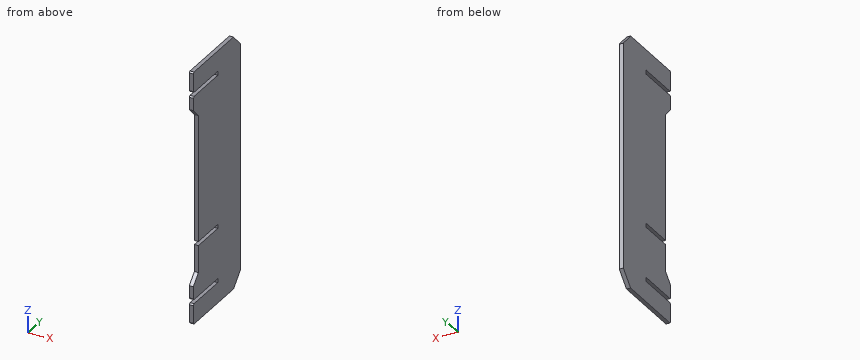
from build123d import *

# Parameters (mm, degrees)
SKETCH1_W                = 3
SKETCH1_H                = 7.073755714
SKETCH1_H_2              = 58.176244286
BOSS_EXTRUDE1_DEPTH      = 15
BOSS_EXTRUDE1_DEPTH_BACK = 171
CUT_EXTRUDE1_REACH       = 5
SKETCH2_W                = 3
SKETCH2_H                = 7.071067812
SKETCH2_H_2              = 26.692349798
CHAMFER1_SIZE            = 10
SKETCH5_W                = 3
SKETCH5_H                = 3
CUT_EXTRUDE2_DEPTH       = 1.002687902
CUT_EXTRUDE3_REACH       = 2.003
SKETCH6_W                = 3
SKETCH6_H                = 3
CHAMFER2_SIZE            = 1


with BuildPart() as part:
    # Sketch1 → Boss-Extrude1 (new body, two sides)
    with BuildSketch(Plane.XY) as boss_extrude1_sk:
        with Locations((-220.627859803, -123.051259948)):
            Rectangle(SKETCH1_W, SKETCH1_H)
        with Locations((-220.627859803, -90.426259948)):
            Rectangle(SKETCH1_W, SKETCH1_H_2)
    extrude(amount=BOSS_EXTRUDE1_DEPTH)
    extrude(boss_extrude1_sk.sketch, amount=-BOSS_EXTRUDE1_DEPTH_BACK)

    # Sketch2 → Cut-Extrude1 (cut, up to next)
    with BuildSketch(Plane(origin=(-219.127859803, 0, 0), x_dir=(0, 0, -1), z_dir=(1, 0, 0)), mode=Mode.PRIVATE) as cut_extrude1_sk1:
        with Locations((1.5, -123.049915997)):
            Rectangle(SKETCH2_W, SKETCH2_H)
    cut_extrude1_tool1 = extrude(cut_extrude1_sk1.sketch, amount=-CUT_EXTRUDE1_REACH, mode=Mode.PRIVATE) & part.part
    add(cut_extrude1_tool1.solids().sort_by_distance((-219.12786, -123.049916, -1.5))[0], mode=Mode.SUBTRACT)
    # Sketch2 → Cut-Extrude1 (cut, up to next)
    with BuildSketch(Plane(origin=(-219.127859803, 0, 0), x_dir=(0, 0, -1), z_dir=(1, 0, 0)), mode=Mode.PRIVATE) as cut_extrude1_sk2:
        with Locations((1.5, -106.168207192)):
            Rectangle(SKETCH2_W, SKETCH2_H_2)
    cut_extrude1_tool2 = extrude(cut_extrude1_sk2.sketch, amount=-CUT_EXTRUDE1_REACH, mode=Mode.PRIVATE) & part.part
    add(cut_extrude1_tool2.solids().sort_by_distance((-219.12786, -106.168207, -1.5))[0], mode=Mode.SUBTRACT)
    # Sketch2 → Cut-Extrude1 (cut, up to next)
    with BuildSketch(Plane(origin=(-219.127859803, 0, 0), x_dir=(0, 0, -1), z_dir=(1, 0, 0)), mode=Mode.PRIVATE) as cut_extrude1_sk3:
        Polygon((116, -126.585449903), (113, -126.585449903), (113, -119.514382091), (20.077559088, -119.514382091), (12.999999639, -126.588137805), (143, -126.588137805), (135.930045977, -119.514382091), (116, -119.514382091), align=None)
    cut_extrude1_tool3 = extrude(cut_extrude1_sk3.sketch, amount=-CUT_EXTRUDE1_REACH, mode=Mode.PRIVATE) & part.part
    add(cut_extrude1_tool3.solids().sort_by_distance((-219.12786, -123.120833, -77.089206))[0], mode=Mode.SUBTRACT)
    # Sketch2 → Cut-Extrude1 (cut, up to next)
    with BuildSketch(Plane(origin=(-219.127859803, 0, 0), x_dir=(0, 0, -1), z_dir=(1, 0, 0)), mode=Mode.PRIVATE) as cut_extrude1_sk4:
        with Locations((114.5, -123.049915997)):
            Rectangle(SKETCH2_W, SKETCH2_H)
    cut_extrude1_tool4 = extrude(cut_extrude1_sk4.sketch, amount=-CUT_EXTRUDE1_REACH, mode=Mode.PRIVATE) & part.part
    add(cut_extrude1_tool4.solids().sort_by_distance((-219.12786, -123.049916, -114.5))[0], mode=Mode.SUBTRACT)
    # Sketch2 → Cut-Extrude1 (cut, up to next)
    with BuildSketch(Plane(origin=(-219.127859803, 0, 0), x_dir=(0, 0, -1), z_dir=(1, 0, 0)), mode=Mode.PRIVATE) as cut_extrude1_sk5:
        with Locations((114.5, -106.168207192)):
            Rectangle(SKETCH2_W, SKETCH2_H_2)
    cut_extrude1_tool5 = extrude(cut_extrude1_sk5.sketch, amount=-CUT_EXTRUDE1_REACH, mode=Mode.PRIVATE) & part.part
    add(cut_extrude1_tool5.solids().sort_by_distance((-219.12786, -106.168207, -114.5))[0], mode=Mode.SUBTRACT)
    # Sketch2 → Cut-Extrude1 (cut, up to next)
    with BuildSketch(Plane(origin=(-219.127859803, 0, 0), x_dir=(0, 0, -1), z_dir=(1, 0, 0)), mode=Mode.PRIVATE) as cut_extrude1_sk6:
        with Locations((154.5, -123.049915997)):
            Rectangle(SKETCH2_W, SKETCH2_H)
    cut_extrude1_tool6 = extrude(cut_extrude1_sk6.sketch, amount=-CUT_EXTRUDE1_REACH, mode=Mode.PRIVATE) & part.part
    add(cut_extrude1_tool6.solids().sort_by_distance((-219.12786, -123.049916, -154.5))[0], mode=Mode.SUBTRACT)
    # Sketch2 → Cut-Extrude1 (cut, up to next)
    with BuildSketch(Plane(origin=(-219.127859803, 0, 0), x_dir=(0, 0, -1), z_dir=(1, 0, 0)), mode=Mode.PRIVATE) as cut_extrude1_sk7:
        with Locations((154.5, -106.168207192)):
            Rectangle(SKETCH2_W, SKETCH2_H_2)
    cut_extrude1_tool7 = extrude(cut_extrude1_sk7.sketch, amount=-CUT_EXTRUDE1_REACH, mode=Mode.PRIVATE) & part.part
    add(cut_extrude1_tool7.solids().sort_by_distance((-219.12786, -106.168207, -154.5))[0], mode=Mode.SUBTRACT)

    # Chamfer1
    chamfer1_edges = [part.edges().sort_by_distance(p)[0] for p in [
        (-220.627859803, -61.338137805, -171),
        (-220.627859803, -61.338137805, 15),
    ]]
    chamfer(chamfer1_edges, length=CHAMFER1_SIZE)

    # Sketch5 → Cut-Extrude2 (cut, through all)
    with BuildSketch(Plane(origin=(0, -126.585449903, 0), x_dir=(1, 0, 0), z_dir=(0, 1, 0))):
        with Locations((-220.627859803, 154.5)):
            Rectangle(SKETCH5_W, SKETCH5_H)
    extrude(amount=-CUT_EXTRUDE2_DEPTH, mode=Mode.SUBTRACT)

    # Sketch6 → Cut-Extrude3 (cut, up to next)
    with BuildSketch(Plane(origin=(0, -126.585449903, 0), x_dir=(1, 0, 0), z_dir=(0, 1, 0)), mode=Mode.PRIVATE) as cut_extrude3_sk1:
        with Locations((-220.627859803, 1.5)):
            Rectangle(SKETCH6_W, SKETCH6_H)
    cut_extrude3_tool1 = extrude(cut_extrude3_sk1.sketch, amount=-CUT_EXTRUDE3_REACH, mode=Mode.PRIVATE) & part.part
    add(cut_extrude3_tool1.solids().sort_by_distance((-220.62786, -126.58545, -1.5))[0], mode=Mode.SUBTRACT)

    # Chamfer2
    chamfer2_edges = [part.edges().sort_by_distance(p)[0] for p in [
        (-220.627859803, -126.588137805, -3),
        (-220.627859803, -126.588137805, 0),
        (-220.627859803, -126.588137805, 15),
        (-220.627859803, -126.588137805, -171),
        (-220.627859803, -126.588137805, -156),
        (-220.627859803, -126.588137805, -153),
    ]]
    chamfer(chamfer2_edges, length=CHAMFER2_SIZE)


solid = part.part
Can you work these out from the model? Positions are in its coordinate system, mm. Coordinates: 2 decimals unless noted, no trailing zeros. Write each loop counter-clockwise with the first axis right and the second up, starting at its lowest first coordinate (ties: lowest second). Pieces come first, ordered by that corner, then holes. Notation, with made-up numbers: (5.5, 73) -> (52.5, 73) arc R16 ccw to (52.5, 81) -> close; hole circle Ø2 at (83, 0.25). An arc over 180 degrees is marked (long way). Write each question's results on one line, items separated by ' | '. Start each with the question number.
Item 1: I'm going to push flat-ended pins straight in: P1, Ø1.5, axis at x = -220.5, z = -72.5, coming from the -Y side; P2, Ø0.9, axis at x = -220, z = -154.5, coming from the -Y side. Where does each tip first touch, or does it pass through?
Item 2: If we section it at B-B, the plane x = -221.6: Write out the boundary of the cut face in (y, z).
Item 3: If we section it at A-A, the plane y = -97.5: Write out the boundary of the cut face in (x, z), and give its area (3 significant figures).
Item 4: If we section it at C-C, the plane z = -42: Write out the boundary of the cut face in (x, y).
Item 5: Please list where these lines run through material, in increasing order: probe 1 along Z at (x, y) = (-219.6, -94); probe 2 along Y at (x, z) = (-219.25, -62); probe 3 along Y at (x, z) = (-219.7, -17.5).
Answer block:
1) P1: y = -119.51 | P2: y = -92.82
2) outline: (-126.59, -170) -> (-125.59, -171) -> (-71.34, -171) -> (-61.34, -161) -> (-61.34, 5) -> (-71.34, 15) -> (-125.59, 15) -> (-126.59, 14) -> (-126.59, 1) -> (-125.59, 0) -> (-92.82, 0) -> (-92.82, -3) -> (-125.59, -3) -> (-126.59, -4) -> (-126.59, -13) -> (-119.51, -20.08) -> (-119.51, -113) -> (-92.82, -113) -> (-92.82, -116) -> (-119.51, -116) -> (-119.51, -135.93) -> (-126.59, -143) -> (-126.59, -152) -> (-125.59, -153) -> (-92.82, -153) -> (-92.82, -156) -> (-125.59, -156) -> (-126.59, -157) -> close
3) outline: (-222.13, -171) -> (-219.13, -171) -> (-219.13, -156) -> (-222.13, -156) -> close; (-222.13, -153) -> (-219.13, -153) -> (-219.13, -116) -> (-222.13, -116) -> close; (-222.13, -113) -> (-219.13, -113) -> (-219.13, -3) -> (-222.13, -3) -> close; (-222.13, 0) -> (-219.13, 0) -> (-219.13, 15) -> (-222.13, 15) -> close | area: 531 mm²
4) outline: (-222.13, -119.51) -> (-219.13, -119.51) -> (-219.13, -61.34) -> (-222.13, -61.34) -> close
5) probe 1: -171 to -156, -153 to -116, -113 to -3, 0 to 15 | probe 2: -119.51 to -61.34 | probe 3: -122.09 to -61.34
